The model under review builds one solid part; all positions refer to its coordinate system, in mm. A direction names the side the tool comes from. Round coordinates to 2 decimals unless told otherwise and drop trailing zeros. Write each loop counter-clockwise with the first axis right and the second up, starting at its lowest first coordinate (ties: lowest second). Pieces come first, ordered by that corner, then holes. Notation, with made-up numbers: (-19.75, -13.75) - (-11.75, -13.75) arc R11 ccw to (-11.75, 1.25) - close; hole circle Ø1 at (50, 23.5). An arc over 180 degrees is marked (long way). Return JSON: item names as keys, results as strings.
from build123d import *

# Parameters (mm, degrees)
SKETCH2_W           = 44
SKETCH2_H           = 29
BOSS_EXTRUDE1_DEPTH = 23
SKETCH3_W           = 40
SKETCH3_H           = 25
CUT_EXTRUDE1_DEPTH  = 21
SKETCH4_W           = 20.7
SKETCH4_H           = 2
CUT_EXTRUDE2_DEPTH  = 33
SKETCH5_W           = 30
SKETCH5_H           = 12.3
CUT_EXTRUDE3_DEPTH  = 2
CUT_EXTRUDE5_DEPTH  = 2
SKETCH11_W          = 3.9
SKETCH11_H          = 8.6
SKETCH11_W_2        = 7
SKETCH11_H_2        = 1.5
CUT_EXTRUDE6_DEPTH  = 2
SKETCH13_W          = 8
SKETCH13_H          = 6
CUT_EXTRUDE8_DEPTH  = 2


with BuildPart() as part:
    # Sketch2 → Boss-Extrude1 (new body)
    with BuildSketch(Plane(origin=(0, 0, 0), x_dir=(1, 0, 0), z_dir=(0, 1, 0))):
        Rectangle(SKETCH2_W, SKETCH2_H)
    extrude(amount=BOSS_EXTRUDE1_DEPTH)

    # Sketch3 → Cut-Extrude1 (cut)
    with BuildSketch(Plane(origin=(0, 23, 0), x_dir=(1, 0, 0), z_dir=(0, 1, 0))):
        Rectangle(SKETCH3_W, SKETCH3_H)
    extrude(amount=-CUT_EXTRUDE1_DEPTH, mode=Mode.SUBTRACT)

    # Sketch4 → Cut-Extrude2 (cut)
    with BuildSketch(Plane.XY.offset(14.5)):
        with Locations((0.25, 18.2)):
            Rectangle(SKETCH4_W, SKETCH4_H)
    extrude(amount=-CUT_EXTRUDE2_DEPTH, mode=Mode.SUBTRACT)

    # Sketch5 → Cut-Extrude3 (cut)
    with BuildSketch(Plane.XY.offset(14.5)):
        with Locations((0, 8.15)):
            Rectangle(SKETCH5_W, SKETCH5_H)
    extrude(amount=-CUT_EXTRUDE3_DEPTH, mode=Mode.SUBTRACT)

    # Sketch8 → Cut-Extrude5 (cut)
    with BuildSketch(Plane(origin=(22, 0, 0), x_dir=(0, 0, -1), z_dir=(1, 0, 0))):
        Polygon((-12.5, 17), (-4, 17), (-4, 13.5), (4, 13.5), (4, 17), (12.5, 17), (12.5, 23), (-12.5, 23), align=None)
    extrude(amount=-CUT_EXTRUDE5_DEPTH, mode=Mode.SUBTRACT)

    # Sketch11 → Cut-Extrude6 (cut)
    with BuildSketch(Plane(origin=(0, 0, -14.5), x_dir=(-1, 0, 0), z_dir=(0, 0, -1))):
        with Locations((-18.05, 6.3)):
            Rectangle(SKETCH11_W, SKETCH11_H)
        with Locations((12.4, 2.75)):
            Rectangle(SKETCH11_W_2, SKETCH11_H_2)
    extrude(amount=-CUT_EXTRUDE6_DEPTH, mode=Mode.SUBTRACT)

    # Sketch13 → Cut-Extrude8 (cut)
    with BuildSketch(Plane(origin=(0, 2, 0), x_dir=(1, 0, 0), z_dir=(0, 1, 0))):
        with Locations((-11, -9.5)):
            Rectangle(SKETCH13_W, SKETCH13_H)
        with Locations((0, -9.5)):
            Rectangle(SKETCH13_W, SKETCH13_H)
        with Locations((11, 9.5)):
            Rectangle(SKETCH13_W, SKETCH13_H)
        with Locations((11, -9.5)):
            Rectangle(SKETCH13_W, SKETCH13_H)
        with Locations((-11, 9.5)):
            Rectangle(SKETCH13_W, SKETCH13_H)
        with Locations((0, 9.5)):
            Rectangle(SKETCH13_W, SKETCH13_H)
    extrude(amount=-CUT_EXTRUDE8_DEPTH, mode=Mode.SUBTRACT)


solid = part.part
(1) For faces 4 (the flat face through (16.1, 6, -14)), 5 (the flat face through (1, 12, -12.5)), 6 (the flat face through (11, 1, 12.5)), 7 (the flat face through (-10.1, 18, 14)), 8 (the flat face through (0, 14.3, 14)), list the 3-axis set-ups (+Z, -Z, +X, -X, +Y, -Y) from which the entire face can be reached by the end or side of a thin tool; tool diameter is ignored.
Filled in:
{"face 4": "-Z", "face 5": "+Y", "face 6": "+Y, -Y", "face 7": "+Z, -Z", "face 8": "+Z"}
(2) Add section D-D (x = -2.5). Write out the cut boundary in (y, z).
Filled in:
{"outline": "(0, -14.5) - (17.2, -14.5) - (17.2, -12.5) - (0, -12.5) - close; (0, -6.5) - (2, -6.5) - (2, 6.5) - (0, 6.5) - close; (0, 12.5) - (2, 12.5) - (2, 14.5) - (0, 14.5) - close; (14.3, 12.5) - (17.2, 12.5) - (17.2, 14.5) - (14.3, 14.5) - close; (19.2, -14.5) - (23, -14.5) - (23, -12.5) - (19.2, -12.5) - close; (19.2, 12.5) - (23, 12.5) - (23, 14.5) - (19.2, 14.5) - close"}
(3) Mouldability with a two-part tool opening along Y and no side actions: class faces 1 (the flat face through (21, 17, -8)), 2 (the flat face through (-15.9, 3, -14)), 3 (the flat face through (-20, 13, 0)) as released by +Y, released by -Y, zero draft, split by the parting line, or undercut.
Filled in:
{"face 1": "released by +Y", "face 2": "undercut", "face 3": "zero draft"}
(4) Wall thickness on line 1 (X direction, y = 11.5, z = -6.25); line 2 (Z direction, x = 18, y = 21); line 3 (X direction, y = 19, z = 11): over which ranges is each line inside the solid? List them lowest first.
Filled in:
{"line 1": "x = -22 to -20, 20 to 22", "line 2": "z = -14.5 to -12.5, 12.5 to 14.5", "line 3": "x = -22 to -20"}
(5) Add section C-C (z = 8.5). Write out the cut boundary in (x, y).
Filled in:
{"outline": "(-22, 0) - (-15, 0) - (-15, 2) - (-20, 2) - (-20, 23) - (-22, 23) - close; (-7, 0) - (-4, 0) - (-4, 2) - (-7, 2) - close; (4, 0) - (7, 0) - (7, 2) - (4, 2) - close; (15, 0) - (22, 0) - (22, 17) - (20, 17) - (20, 2) - (15, 2) - close"}
(6) Add section B-B (x = 12). Write out the cut boundary in (y, z), plus the area to 3 significant figures.
Filled in:
{"outline": "(0, -14.5) - (23, -14.5) - (23, -12.5) - (0, -12.5) - close; (0, -6.5) - (2, -6.5) - (2, 6.5) - (0, 6.5) - close; (0, 12.5) - (2, 12.5) - (2, 14.5) - (0, 14.5) - close; (14.3, 12.5) - (23, 12.5) - (23, 14.5) - (14.3, 14.5) - close", "area": "93.4 mm2"}
(7) Add section A-A (y = 8). Write out the cut boundary in (x, z).
Filled in:
{"outline": "(-22, -14.5) - (16.1, -14.5) - (16.1, -12.5) - (-20, -12.5) - (-20, 12.5) - (-15, 12.5) - (-15, 14.5) - (-22, 14.5) - close; (15, 12.5) - (20, 12.5) - (20, -14.5) - (22, -14.5) - (22, 14.5) - (15, 14.5) - close"}
